from build123d import *

# Parameters (mm, degrees)
F0_R            = 1.5875
F1_DEPTH        = 1.5875
F2_R            = 1.0922
F3_DEPTH        = 1.5875
F3_COPIES_COUNT = 3
F4_R            = 4.7625


# Not quite as in the source:
# - a pattern or mirror of a feature is missing from the dataset's text; its kind, count and spacing are read off the source's solid


with BuildPart() as f1:
    # F0 (on Top) → F1 (new body)
    with BuildSketch(Plane.XY):
        Polygon((65.9911357684, -38.1), (65.9911357684, 38.1), (0, 76.2), (-65.9911357684, 38.1), (-65.9911357684, -38.1), (0, -76.2), align=None)
        with Locations((-35.1536, -35.1536)):
            Circle(F0_R, mode=Mode.SUBTRACT)
        with Locations((35.1536, -35.1536)):
            Circle(F0_R, mode=Mode.SUBTRACT)
        with Locations((-35.1536, 35.1536)):
            Circle(F0_R, mode=Mode.SUBTRACT)
        with Locations((35.1536, 35.1536)):
            Circle(F0_R, mode=Mode.SUBTRACT)
    extrude(amount=F1_DEPTH)

    # F2 (on face) → F3 (cut, through all)
    with BuildSketch(Plane.XY.offset(1.5875)):
        with BuildLine():
            ThreePointArc((11.8486437632, -13.2566225326), (0, -17.78), (-11.8486437632, -13.2566225326))
            ThreePointArc((-11.8486437632, -13.2566225326), (-14.3916795622, -13.9960432527), (-16.9881251543, -13.4742728402))
            Line((-16.9881251543, -13.4742728402), (-31.2933003438, -21.7333695867))
            ThreePointArc((-31.2933003438, -21.7333695867), (0, -38.1), (31.2933003438, -21.7333695867))
            Line((31.2933003438, -21.7333695867), (16.9881251543, -13.4742728402))
            ThreePointArc((16.9881251543, -13.4742728402), (14.3916795622, -13.9960432527), (11.8486437632, -13.2566225326))
        make_face()
        with Locations((14.6267687632, -8.4447688828)):
            Circle(F2_R)
        with Locations((-14.6267687632, -8.4447688828)):
            Circle(F2_R)
    f3 = extrude(amount=-F3_DEPTH, mode=Mode.SUBTRACT)

    # F3_copies: F3 ×3 about axis
    f3_copies_axis = Axis((0, 0, 0), (0, 0, 1))
    for i in range(1, F3_COPIES_COUNT):
        add(f3.rotate(f3_copies_axis, i * 360 / F3_COPIES_COUNT), mode=Mode.SUBTRACT)

    # F4
    f4_edges = [f1.edges().sort_by_distance(p)[0] for p in [
        (-65.991136, 38.1, 0.79375),
        (0, 76.2, 0.79375),
        (65.991136, 38.1, 0.79375),
        (65.991136, -38.1, 0.79375),
        (0, -76.2, 0.79375),
        (-65.991136, -38.1, 0.79375),
    ]]
    fillet(f4_edges, radius=F4_R)


solid = f1.part
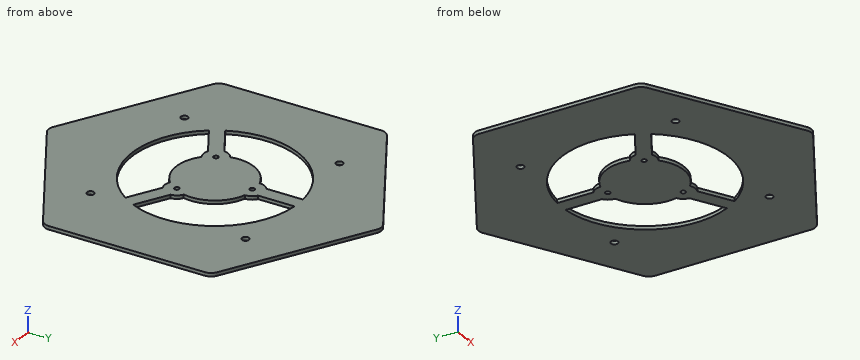
Design review of the part built by this model. Coordinates are the model's own, in mm. Coordinates: 2 decimals unless noted, no trailing zeros. Loops run counter-clockwise (first coordinate to the right, second up) from the corner with the lowest first, then second, coordinate; pieces in that order, holes last. Notation, with made-up numbers: (46, -1.5) - (85, -1.5) arc R25 ccw to (85, 15.5) - close; hole circle Ø6 at (-3.5, -6). An arc over 180 degrees is marked (long way). Use CSV: the item, a comma, the result in double quotes. Start each with the question number.
1. Add section C-C on y = -31. Give the boundary of the cut face in (x, z), plus the area to 3 significant figures.
2. Add section D-D on z = 0.7. Count the separate pieces of the cut face and the enclosed holes in it, plus the area to 3 significant figures.
3. To check wall thickness, follow probe 1 along Y at (x, z) = (0, 0.8); probe 2 along Y at (x, z) = (-6, 1.2); probe 3 along X at (y, z) = (13.5, 1.1). State the ranges of each line that lie inside material, in increasing order.
4. Add section B-B on x = 29. Give the boundary of the cut face in (y, z), plus the area to 3 significant figures.
5. Add section A-A on y = 13. Give the boundary of the cut face in (x, z), plus the area to 3 significant figures.
Resolved:
1,outline,"(-65.99, 0) - (-22.15, 0) - (-22.15, 1.59) - (-65.99, 1.59) - close; (22.15, 0) - (65.99, 0) - (65.99, 1.59) - (22.15, 1.59) - close"
1,area,"139 mm2"
2,separate pieces,"1"
2,enclosed holes,"10"
2,area,"11,900 mm2"
3,probe 1,"-75.46 to -38.1, -17.78 to 15.8, 17.98 to 75.46"
3,probe 2,"-72.74 to -37.62, -16.74 to 16.74, 37.62 to 72.74"
3,probe 3,"-65.99 to -35.63, -11.57 to 11.57, 35.63 to 65.99"
4,outline,"(-59.46, 0) - (-24.71, 0) - (-24.71, 1.59) - (-59.46, 1.59) - close; (-20.41, 0) - (-13.08, 0) - (-13.08, 1.59) - (-20.41, 1.59) - close; (24.71, 0) - (59.46, 0) - (59.46, 1.59) - (24.71, 1.59) - close"
4,area,"122 mm2"
5,outline,"(-65.99, 0) - (-35.81, 0) - (-35.81, 1.59) - (-65.99, 1.59) - close; (-12.13, 0) - (12.13, 0) - (12.13, 1.59) - (-12.13, 1.59) - close; (35.81, 0) - (65.99, 0) - (65.99, 1.59) - (35.81, 1.59) - close"
5,area,"134 mm2"
